```python
from build123d import *

# Parameters (mm, degrees)
ESQUISSE1_W             = 24
ESQUISSE1_H             = 28
BOSS_EXTRU_1_DEPTH      = 24
ENL_V_MAT_EXTRU_1_DEPTH = 24
ESQUISSE5_W             = 24
ESQUISSE5_H             = 24
BOSS_EXTRU_2_DEPTH      = 5
ENL_V_MAT_EXTRU_6_DEPTH = 24
ESQUISSE7_R             = 1.75
ENL_V_MAT_EXTRU_8_DEPTH = 5


with BuildPart() as part:
    # Esquisse1 → Boss.-Extru.1 (new body)
    with BuildSketch(Plane(origin=(0, 0, 0), x_dir=(1, 0, 0), z_dir=(0, 1, 0))):
        Rectangle(ESQUISSE1_W, ESQUISSE1_H)
    extrude(amount=BOSS_EXTRU_1_DEPTH)

    # Esquisse3 → Enlèv. mat.-Extru.1 (cut)
    with BuildSketch(Plane(origin=(0, 24, 0), x_dir=(1, 0, 0), z_dir=(0, 1, 0))):
        Polygon((-10, -12), (-2.45, -12), (-2.45, -10.45), (-6.15, -10.45), (-6.15, -9.45), (-2.645559959, -5.8), (2.645559959, -5.8), (6.15, -9.45), (6.15, -10.45), (2.45, -10.45), (2.45, -12), (10, -12), (10, -4.45), (8.45, -4.45), (8.45, -8.15), (7.45, -8.15), (3.8, -4.654440041), (3.8, 0.645559959), (7.45, 4.15), (8.45, 4.15), (8.45, 0.45), (10, 0.45), (10, 8), (2.45, 8), (2.45, 6.45), (6.15, 6.45), (6.15, 5.45), (2.645559959, 1.8), (-2.645559959, 1.8), (-6.15, 5.45), (-6.15, 6.45), (-2.45, 6.45), (-2.45, 8), (-10, 8), (-10, 0.45), (-8.45, 0.45), (-8.45, 4.15), (-7.45, 4.15), (-3.8, 0.654440041), (-3.8, -4.645559959), (-7.45, -8.15), (-8.45, -8.15), (-8.45, -4.45), (-10, -4.45), align=None)
    extrude(amount=-ENL_V_MAT_EXTRU_1_DEPTH, mode=Mode.SUBTRACT)

    # Esquisse5 → Boss.-Extru.2 (add)
    with BuildSketch(Plane(origin=(0, 0, -14), x_dir=(-1, 0, 0), z_dir=(0, 0, -1))):
        with Locations((0, 12)):
            Rectangle(ESQUISSE5_W, ESQUISSE5_H)
    extrude(amount=BOSS_EXTRU_2_DEPTH)

    # Esquisse6 → Enlèv. mat.-Extru.6 (cut)
    with BuildSketch(Plane(origin=(0, 24, 0), x_dir=(1, 0, 0), z_dir=(0, 1, 0))):
        Polygon((-10, 8), (-10, 14), (10, 14), (10, 8), (2.45, 8), (2.45, 6.45), (6.15, 6.45), (6.15, 5.45), (2.645559959, 1.8), (-2.645559959, 1.8), (-6.15, 5.45), (-6.15, 6.45), (-2.45, 6.45), (-2.45, 8), align=None)
    extrude(amount=-ENL_V_MAT_EXTRU_6_DEPTH, mode=Mode.SUBTRACT)

    # Esquisse7 → Enlèv. mat.-Extru.8 (cut)
    with BuildSketch(Plane(origin=(0, 0, -19), x_dir=(-1, 0, 0), z_dir=(0, 0, -1))):
        with Locations((-6, 18)):
            Circle(ESQUISSE7_R)
        with Locations((-6, 6)):
            Circle(ESQUISSE7_R)
        with Locations((6, 6)):
            Circle(ESQUISSE7_R)
        with Locations((6, 18)):
            Circle(ESQUISSE7_R)
    extrude(amount=-ENL_V_MAT_EXTRU_8_DEPTH, mode=Mode.SUBTRACT)


solid = part.part
```
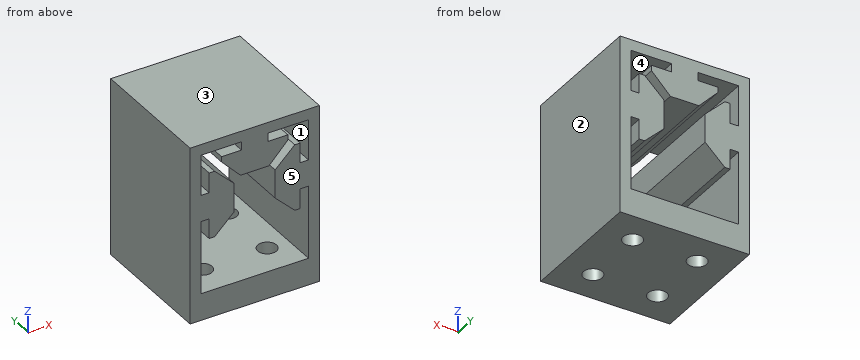
For this review, take the finished solid that the model builds, in its own axes (mm). Face numbers are marked on the shaded views. A direction names the side the tool comes from. Coordinates: 2 decimals unless noted, no trailing zeros. Loops run counter-clockwise (first coordinate to the right, second up) from the corner with the lowest first, then second, coordinate; pieces in that order, holes last. Notation, with made-up numbers: (7, 59.25) -> (17, 59.25) arc R21 ccw to (17, 65.25) -> close; hole circle Ø7 at (80.25, 58.25). An arc over 180 degrees is marked (long way). Return JSON: item names as keys, results as strings. Group by question number.
(1) Mouldability with a two-part tool opening along X and no side actions: class the marked faces 1, 2 and 3 as pulls with the +X half, pulls with the -X half, needs draft (parallel to the pull), parting line crosses it, or undercut.
(2) For pin 1 Ø3 at (x, y) = (6, 6) entering from -Z, flat-tipped, find the tip position at first contact; note if it passes through.
(3) Tool access review of the marked faces 4 and 5: name each direction out of +Z, -Z, +X, -X, +Y, -Y from which nothing blocks a thin tool from reaching the whole face with its end or side.
(4) To check wall thickness, follow L1, parallel to Y at x = 6, z = -16; L2, parallel to Z at x = 2.5, y = 11.75; L3, parallel to Z at x = 8.5, y = 13.5. State the ranges of each line that lie inside material, in increasing order.
(5) Consider section B-B, the plane z = -11. Give the boundary of the cut face in (x, y).
(6) Consider section A-A, the plane x = -0.25. Give the boundary of the cut face in (y, z).
Results below:
{
 "1": {"face 1": "undercut", "face 2": "pulls with the +X half", "face 3": "needs draft"},
 "2": {"pin 1": "stops at z = -4.15"},
 "3": {"face 4": "+Y, -Y", "face 5": "+Z, -Z, +X, -X, -Y"},
 "4": {"L1": "y = 0 to 4.25, 7.75 to 16.25, 19.75 to 24", "L2": "z = -19 to -14, 5.8 to 10.45, 12 to 14", "L3": "z = -19 to -14, -0.45 to 4.45, 12 to 14"},
 "5": {"outline": "(-12, 0) -> (-10, 0) -> (-10, 24) -> (-12, 24) -> close; (10, 0) -> (12, 0) -> (12, 24) -> (10, 24) -> close"},
 "6": {"outline": "(0, -19) -> (24, -19) -> (24, -14) -> (0, -14) -> close; (0, 5.8) -> (24, 5.8) -> (24, 14) -> (0, 14) -> close"}
}
